Could you check a few things on this model? Use its own coordinates, in mm. Face numbers are marked on the shaded views. A direction names the side the tool comes from. Round coordinates to 2 decimals unless told otherwise and drop trailing zeros. Write each loop counter-clockwise with the first axis right and the second up, starting at its lowest first coordinate (ties: lowest second). Pieces come first, ordered by that corner, then holes. Notation, with made-up numbers: (-11, 23.5) -> (33, 23.5) arc R27 cw to (33, 53.5) -> close; hole circle Ø8 at (29.5, -32.5). An arc over 180 degrees is marked (long way). Return JSON: item names as keys, results as strings.
from build123d import *
from build123d.topology import SkipClean

# Parameters (mm, degrees)
SKETCH1_R           = 55
BOSS_EXTRUDE1_DEPTH = 5
SKETCH2_W           = 30
SKETCH2_H           = 14
BOSS_EXTRUDE2_DEPTH = 30
SKETCH6_R           = 2.05
CUT_EXTRUDE3_DEPTH  = 30
SKETCH7_W           = 30
SKETCH7_H           = 3.4
CUT_EXTRUDE4_DEPTH  = 6
SKETCH8_R           = 5
BOSS_EXTRUDE3_DEPTH = 30
CIRPATTERN1_COUNT   = 2
SKETCH9_R           = 55
SKETCH9_R_2         = 45
BOSS_EXTRUDE4_DEPTH = 5
SKETCH10_R          = 1.6
CUT_EXTRUDE5_DEPTH  = 6
SKETCH11_W          = 30
SKETCH11_H          = 17.3
CUT_EXTRUDE6_DEPTH  = 1.5
BOSS_EXTRUDE5_DEPTH = 5
SKETCH16_R          = 4
BOSS_EXTRUDE6_DEPTH = 5
SKETCH17_R          = 1.6
CUT_EXTRUDE8_DEPTH  = 98.724101428
SKETCH13_R          = 5
CUT_EXTRUDE9_DEPTH  = 2
CIRPATTERN3_COUNT   = 4
FILLET1_R           = 2


with BuildPart() as part:
    # Sketch1 → Boss-Extrude1 (new body)
    with BuildSketch(Plane(origin=(0, 0, 0), x_dir=(1, 0, 0), z_dir=(0, 1, 0))):
        with Locations(Location((0, 0, 0), (0, 0, 270))):
            Circle(SKETCH1_R)
    extrude(amount=BOSS_EXTRUDE1_DEPTH)

    # Sketch2 → Boss-Extrude2 (add)
    with BuildSketch(Plane(origin=(0, 5, 0), x_dir=(1, 0, 0), z_dir=(0, 1, 0))):
        with Locations((0, -27.9)):
            Rectangle(SKETCH2_W, SKETCH2_H)
    extrude(amount=BOSS_EXTRUDE2_DEPTH)

    # Sketch6 → Cut-Extrude3 (cut)
    with BuildSketch(Plane(origin=(0, 35, 0), x_dir=(1, 0, 0), z_dir=(0, 1, 0))):
        with Locations(Location((-6, -24, 0), (0, 0, 270))):
            Circle(SKETCH6_R)
        with Locations(Location((0, -24, 0), (0, 0, 270))):
            Circle(SKETCH6_R)
        with Locations(Location((6, -24, 0), (0, 0, 270))):
            Circle(SKETCH6_R)
    extrude(amount=-CUT_EXTRUDE3_DEPTH, mode=Mode.SUBTRACT)

    # Sketch7 → Cut-Extrude4 (cut)
    with BuildSketch(Plane(origin=(0, 0, 20.9), x_dir=(-1, 0, 0), z_dir=(0, 0, -1))):
        with Locations((0, 6.7)):
            Rectangle(SKETCH7_W, SKETCH7_H)
        with Locations((0, 27.4)):
            Rectangle(SKETCH7_W, SKETCH7_H)
    extrude(amount=-CUT_EXTRUDE4_DEPTH, mode=Mode.SUBTRACT)

    # Sketch8 → Boss-Extrude3 (add)
    with BuildSketch(Plane(origin=(0, 5, 0), x_dir=(1, 0, 0), z_dir=(0, 1, 0))):
        with Locations(Location((-50, 0, 0), (0, 0, 180))):
            Circle(SKETCH8_R)
    boss_extrude3 = extrude(amount=BOSS_EXTRUDE3_DEPTH)

    # CirPattern1: Boss-Extrude3 ×2 about axis
    cirpattern1_axis = Axis((0, 0, 0), (0, 1, 0))
    for i in range(1, CIRPATTERN1_COUNT):
        add(boss_extrude3.rotate(cirpattern1_axis, i * 360 / CIRPATTERN1_COUNT))

    # Sketch9 → Boss-Extrude4 (add)
    with BuildSketch(Plane(origin=(0, 35, 0), x_dir=(1, 0, 0), z_dir=(0, 1, 0))):
        with Locations(Location((0, 0, 0), (0, 0, 3.4551e-05))):
            Circle(SKETCH9_R)
        Circle(SKETCH9_R_2, mode=Mode.SUBTRACT)
    extrude(amount=BOSS_EXTRUDE4_DEPTH)

    # Sketch10 → Cut-Extrude5 (cut)
    with BuildSketch(Plane.XZ):
        with Locations(Location((-28.284271247, 28.284271247, 0), (0, 0, 270))):
            Circle(SKETCH10_R)
        with Locations(Location((28.284271247, 28.284271247, 0), (0, 0, 270))):
            Circle(SKETCH10_R)
        with Locations(Location((28.284271247, -28.284271247, 0), (0, 0, 270))):
            Circle(SKETCH10_R)
        with Locations(Location((-28.284271247, -28.284271247, 0), (0, 0, 270))):
            Circle(SKETCH10_R)
    extrude(amount=-CUT_EXTRUDE5_DEPTH, mode=Mode.SUBTRACT)

    # Sketch11 → Cut-Extrude6 (cut)
    with BuildSketch(Plane(origin=(0, 0, 20.9), x_dir=(-1, 0, 0), z_dir=(0, 0, -1))):
        with Locations((0, 17.05)):
            Rectangle(SKETCH11_W, SKETCH11_H)
    extrude(amount=-CUT_EXTRUDE6_DEPTH, mode=Mode.SUBTRACT)

    # Sketch14 → Boss-Extrude5 (add)
    with SkipClean():  # the faces are left unmerged after this step: merging them gives an invalid solid
        with BuildSketch(Plane.XZ):
            Polygon((-26, -48.466483264), (-26, -75), (26, -75), (26, -25), (-26, -25), align=None)
        extrude(amount=-BOSS_EXTRUDE5_DEPTH)

    # Sketch16 → Boss-Extrude6 (add)
    with BuildSketch(Plane(origin=(0, 5, 0), x_dir=(1, 0, 0), z_dir=(0, 1, 0))):
        with Locations(Location((-21, 68, 0), (0, 0, 270))):
            Circle(SKETCH16_R)
        with Locations(Location((21.07, 68, 0), (0, 0, 270))):
            Circle(SKETCH16_R)
        with Locations(Location((-21, 19.96, 0), (0, 0, 270))):
            Circle(SKETCH16_R)
        with Locations(Location((21.07, 19.96, 0), (0, 0, 270))):
            Circle(SKETCH16_R)
    extrude(amount=BOSS_EXTRUDE6_DEPTH)

    # Sketch17 → Cut-Extrude8 (cut, through all)
    with BuildSketch(Plane(origin=(0, 10, 0), x_dir=(1, 0, 0), z_dir=(0, 1, 0))):
        with Locations(Location((-21, 68, 0), (0, 0, 270))):
            Circle(SKETCH17_R)
        with Locations(Location((21.07, 68, 0), (0, 0, 270))):
            Circle(SKETCH17_R)
        with Locations(Location((21.07, 19.96, 0), (0, 0, 270))):
            Circle(SKETCH17_R)
        with Locations(Location((-21, 19.96, 0), (0, 0, 270))):
            Circle(SKETCH17_R)
    extrude(amount=-CUT_EXTRUDE8_DEPTH, mode=Mode.SUBTRACT)

    # Sketch13 → Cut-Extrude9 (cut)
    with BuildSketch(Plane(origin=(0, 5, 0), x_dir=(1, 0, 0), z_dir=(0, 1, 0))):
        with Locations(Location((-28.284271247, 28.284271247, 0), (0, 0, 270))):
            Circle(SKETCH13_R)
    cut_extrude9 = extrude(amount=-CUT_EXTRUDE9_DEPTH, mode=Mode.SUBTRACT)

    # CirPattern3: Cut-Extrude9 ×4 about axis
    cirpattern3_axis = Axis((0, 0, 0), (0, 1, 0))
    for i in range(1, CIRPATTERN3_COUNT):
        add(cut_extrude9.rotate(cirpattern3_axis, i * 360 / CIRPATTERN3_COUNT), mode=Mode.SUBTRACT)

    # Fillet1
    fillet1_edges = [part.edges().sort_by_distance(p)[0] for p in [
        (-55, 40, 3.3167e-05),
        (-45, 40, 0),
    ]]
    fillet(fillet1_edges, radius=FILLET1_R)


solid = part.part
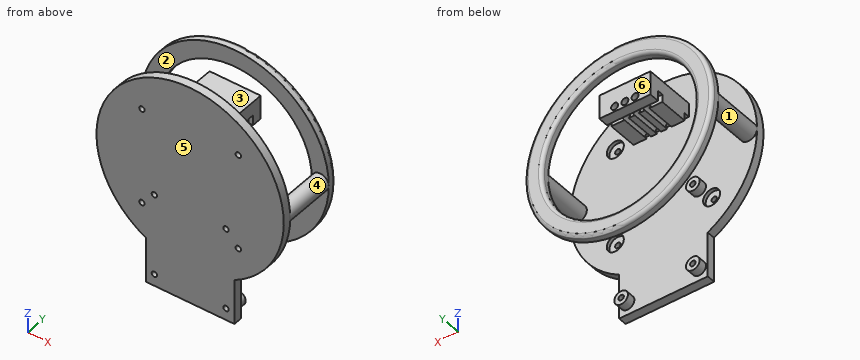
1) I want a section at A-A, the plane y = 17.5. Please give me the cut outline in (x, z).
Return value:
{"outline": "circle Ø10 at (-50, 0); (-15, 22.4) -> (-7.28, 22.4) arc R2.05 cw (long way) to (-4.72, 22.4) -> (-1.28, 22.4) arc R2.05 cw (long way) to (1.28, 22.4) -> (4.72, 22.4) arc R2.05 cw (long way) to (7.28, 22.4) -> (15, 22.4) -> (15, 34.9) -> (-15, 34.9) -> close; circle Ø10 at (50, 0)"}
2) Thinking about a two-plate mould opening in Z: for the marked faces 4, 5 and 6, which applies, pulls with the +Z half, pulls with the -Z half, needs draft (parallel to the pull), parting line crosses it, or undercut?
Return value:
{"face 4": "parting line crosses it", "face 5": "needs draft", "face 6": "undercut"}
3) For the marked faces 1, 2 and 3, which set-ups out of +Z, -Z, +X, -X, +Y, -Y let a thin tool reach every point of the face, with its end or its side?
Return value:
{"face 1": "none", "face 2": "+Z", "face 3": "+Z, +X, -X, +Y"}
4) If I drill on probe 1 along Y at (x, z) = (-12.5, 25); probe 2 along Z at (x, y) = (0, 36.55); probe 3 along Y at (x, z) = (49, 7), over which ranges is the centre line in solid material (lowest first)? Write a range as [from, to].
Return value:
{"probe 1": "[0, 5], [8.4, 25.7], [29.1, 35]", "probe 2": "[-55, -45], [45, 55]", "probe 3": "[0, 5], [35, 40]"}
5) I want a section at C-C, the plane x = -21. Count the separate pieces of the cut face and the enclosed holes in it, and give its area (3 significant figures).
Return value:
{"separate pieces": "5", "enclosed holes": "0", "area": "752 mm²"}
6) Will these pins go through, and if not, where does the flat tip stop? pin 1 Ø6 at (x, y) = (10.5, 18) entering from -Z; pin 2 Ø6 at (x, z) = (42.5, 1) entering from -Y; pin 3 Ø6 at (y, z) = (15, -26.5) entering from +X; pin 4 Ø10 at (x, y) = (-28, 8.5) entering from +Z.
Return value:
{"pin 1": "z = 22.4", "pin 2": "y = 0", "pin 3": "through", "pin 4": "z = 49.28"}
7) I want a section at B-B, the plane z = -68. Please give me the cut outline in (x, y), and give its area (3 significant figures).
Return value:
{"outline": "(-26, 0) -> (-22.6, 0) -> (-22.6, 10) -> (-25, 10) -> (-25, 5) -> (-26, 5) -> close; (-19.4, 0) -> (19.47, 0) -> (19.47, 10) -> (17.07, 10) -> (17.07, 5) -> (-17, 5) -> (-17, 10) -> (-19.4, 10) -> close; (22.67, 0) -> (26, 0) -> (26, 5) -> (25.07, 5) -> (25.07, 10) -> (22.67, 10) -> close", "area": "276 mm²"}
